Here's how the part is built. I have some questions about the finished solid (model axes, mm). A direction names the side the tool comes from. Coordinates: 2 decimals unless noted, no trailing zeros. Write each loop counter-clockwise with the first axis right and the second up, starting at its lowest first coordinate (ties: lowest second). Pieces come first, ordered by that corner, then holes.
(1) Thinking about a two-plate mould opening in Z: for faces 1 (the flat face through (5, -28, 18)), 2 (the cylindrical face through (9.9, -75, 0.5)), 3 (the flat face through (30, 1, 1)), which applies, released by +Z, released by -Z, zero draft, split by the parting line, or undercut?
(2) Imagine slicing it at A-A, the plane z = 0. List the corners of the cut face in (x, y) for me, plus the area to 3 significant figures.
(3) Imagine slicing it at B-B, the plane x = 27.25. List the corners of the cut face in (y, z) for me, plus the area to 3 significant figures.
(4) For pin 1 Ø10 at (x, z) = (10.5, 45.5) entering from +Y; pin 2 Ø9.5 at (x, z) = (11.5, -34.5) entering from +Y; pin 3 Ø7 at (y, z) = (2.5, 36) entering from +X; pin 4 Ø9 at (y, z) = (-58, 0) entering from -X, each with a flat end and sliding along its axis, tell me the tip position at first contact or that it passes through.
(5) Imagine slicing it at C-C, the plane x = 2. List the corners of the cut face in (y, z) for me, plus the area to 3 significant figures.
(6) Which directions (+Z, -Z, +X, -X, +Y, -Y) give clear straight access to the entire face, cutting with the end or side of a thin tool? Please do faces 4 (the cylindrical face through (9.86, -59.44, 32.58)), 5 (the cylindrical face through (19.86, 20.17, 34.54)), 6 (the cylindrical face through (25, -40, 0)), 7 (the flat face through (17, -7, -31)).
(7) Please list where these lines run through material, in increasing order: probe 1 along Y at (x, z) = (12.25, 0); probe 2 along Y at (x, z) = (8.25, 34.5); probe 3 along Y at (x, z) = (8, -31.5).
(8) Imagine slicing it at D-D, the plane z = -31.5. List the corners of the cut face in (x, y) for me, plus the area to 3 significant figures.
```python
from build123d import *

# Parameters (mm, degrees)
BOSS_EXTRUDE1_DEPTH                             = 10
BOSS_EXTRUDE1_2_DEPTH                           = 10
BOSS_EXTRUDE2_DEPTH                             = 30
BOSS_EXTRUDE3_DEPTH                             = 5
SKETCH1_5_R                                     = 5
BOSS_EXTRUDE4_DEPTH                             = 20
CSK_FOR_M8_FLAT_HEAD_MACHINE_SCREW1_D           = 10
CSK_FOR_M8_FLAT_HEAD_MACHINE_SCREW1_CSINK_D     = 17.3
CSK_FOR_M8_FLAT_HEAD_MACHINE_SCREW1_CSINK_ANGLE = 90


with BuildPart() as part:
    # Sketch1 → Boss-Extrude1 (new body)
    with BuildSketch(Plane(origin=(0, 0, 0), x_dir=(0, 0, -1), z_dir=(1, 0, 0))):
        with BuildLine():
            ThreePointArc((-26.062177826, 31.141016151), (-26.761480784, 36.452749467), (-23.5, 40.703193978))
            Line((-23.5, 40.703193978), (-25.5, 44.167295593))
            ThreePointArc((-25.5, 44.167295593), (-35.403493203, 43.212233307), (-42.62357008, 50.057802056))
            ThreePointArc((-42.62357008, 50.057802056), (-42.094968285, 33.486802939), (-52.43535512, 20.527102646))
            ThreePointArc((-52.43535512, 20.527102646), (-64, 0), (-52.43535512, -20.527102646))
            ThreePointArc((-52.43535512, -20.527102646), (-42.094968285, -33.486802939), (-42.62357008, -50.057802056))
            ThreePointArc((-42.62357008, -50.057802056), (-35.403493203, -43.212233307), (-25.5, -44.167295593))
            Line((-25.5, -44.167295593), (-23.5, -40.703193978))
            ThreePointArc((-23.5, -40.703193978), (-26.761480784, -36.452749467), (-26.062177826, -31.141016151))
            Line((-26.062177826, -31.141016151), (-25.753546494, -30.606451003))
            ThreePointArc((-25.753546494, -30.606451003), (-34.641016151, -20), (-39.382737335, -7))
            Line((-39.382737335, -7), (-40, -7))
            ThreePointArc((-40, -7), (-47, 0), (-40, 7))
            Line((-40, 7), (-39.382737335, 7))
            ThreePointArc((-39.382737335, 7), (-34.641016151, 20), (-25.753546494, 30.606451003))
            Line((-25.753546494, 30.606451003), (-26.062177826, 31.141016151))
        make_face()
    extrude(amount=BOSS_EXTRUDE1_DEPTH)



with BuildPart() as body_2:
    # Sketch1 → Boss-Extrude1 2 (new body)
    with BuildSketch(Plane(origin=(0, 0, 0), x_dir=(0, 0, -1), z_dir=(1, 0, 0))):
        with BuildLine():
            ThreePointArc((25.753546494, 30.606451003), (34.641016151, 20), (39.382737335, 7))
            Line((39.382737335, 7), (40, 7))
            ThreePointArc((40, 7), (47, 0), (40, -7))
            Line((40, -7), (39.382737335, -7))
            ThreePointArc((39.382737335, -7), (34.641016151, -20), (25.753546494, -30.606451003))
            Line((25.753546494, -30.606451003), (26.062177826, -31.141016151))
            ThreePointArc((26.062177826, -31.141016151), (26.761480784, -36.452749467), (23.5, -40.703193978))
            Line((23.5, -40.703193978), (25.5, -44.167295593))
            ThreePointArc((25.5, -44.167295593), (35.403493203, -43.212233307), (42.62357008, -50.057802056))
            ThreePointArc((42.62357008, -50.057802056), (42.094968285, -33.486802939), (52.43535512, -20.527102646))
            ThreePointArc((52.43535512, -20.527102646), (64, 0), (52.43535512, 20.527102646))
            ThreePointArc((52.43535512, 20.527102646), (42.094968285, 33.486802939), (42.62357008, 50.057802056))
            ThreePointArc((42.62357008, 50.057802056), (35.403493203, 43.212233307), (25.5, 44.167295593))
            Line((25.5, 44.167295593), (23.5, 40.703193978))
            ThreePointArc((23.5, 40.703193978), (26.761480784, 36.452749467), (26.062177826, 31.141016151))
            Line((26.062177826, 31.141016151), (25.753546494, 30.606451003))
        make_face()
    extrude(amount=BOSS_EXTRUDE1_2_DEPTH)


with BuildPart() as part_1:
    add(part.part)

    add(body_2.part)  # Boss-Extrude2 merges body 2
    # Sketch1_3 → Boss-Extrude2 (add)
    with BuildSketch(Plane(origin=(0, 0, 0), x_dir=(0, 0, -1), z_dir=(1, 0, 0))):
        with BuildLine():
            Line((21, -7), (21, 7))
            Line((21, 7), (39.382737335, 7))
            ThreePointArc((39.382737335, 7), (34.641016151, 20), (25.753546494, 30.606451003))
            Line((25.753546494, 30.606451003), (16.562177826, 14.686533479))
            Line((16.562177826, 14.686533479), (4.437822174, 21.686533479))
            Line((4.437822174, 21.686533479), (13.629190841, 37.606451003))
            ThreePointArc((13.629190841, 37.606451003), (0, 40), (-13.629190841, 37.606451003))
            Line((-13.629190841, 37.606451003), (-4.437822174, 21.686533479))
            Line((-4.437822174, 21.686533479), (-16.562177826, 14.686533479))
            Line((-16.562177826, 14.686533479), (-25.753546494, 30.606451003))
            ThreePointArc((-25.753546494, 30.606451003), (-34.641016151, 20), (-39.382737335, 7))
            Line((-39.382737335, 7), (-21, 7))
            Line((-21, 7), (-21, -7))
            Line((-21, -7), (-39.382737335, -7))
            ThreePointArc((-39.382737335, -7), (-34.641016151, -20), (-25.753546494, -30.606451003))
            Line((-25.753546494, -30.606451003), (-16.562177826, -14.686533479))
            Line((-16.562177826, -14.686533479), (-4.437822174, -21.686533479))
            Line((-4.437822174, -21.686533479), (-13.629190841, -37.606451003))
            ThreePointArc((-13.629190841, -37.606451003), (0, -40), (13.629190841, -37.606451003))
            Line((13.629190841, -37.606451003), (4.437822174, -21.686533479))
            Line((4.437822174, -21.686533479), (16.562177826, -14.686533479))
            Line((16.562177826, -14.686533479), (25.753546494, -30.606451003))
            ThreePointArc((25.753546494, -30.606451003), (34.641016151, -20), (39.382737335, -7))
            Line((39.382737335, -7), (21, -7))
        make_face()
    extrude(amount=BOSS_EXTRUDE2_DEPTH)

    # Sketch1_4 → Boss-Extrude3 (add)
    with BuildSketch(Plane(origin=(0, 0, 0), x_dir=(0, 0, -1), z_dir=(1, 0, 0))):
        with BuildLine():
            ThreePointArc((13.937822174, 38.141016151), (23.5, 40.703193978), (26.062177826, 31.141016151))
            Line((26.062177826, 31.141016151), (16.562177826, 14.686533479))
            Line((16.562177826, 14.686533479), (4.437822174, 21.686533479))
            Line((4.437822174, 21.686533479), (13.937822174, 38.141016151))
        make_face()
        with BuildLine():
            ThreePointArc((-26.062177826, 31.141016151), (-23.5, 40.703193978), (-13.937822174, 38.141016151))
            Line((-13.937822174, 38.141016151), (-4.437822174, 21.686533479))
            Line((-4.437822174, 21.686533479), (-16.562177826, 14.686533479))
            Line((-16.562177826, 14.686533479), (-26.062177826, 31.141016151))
        make_face()
        with BuildLine():
            ThreePointArc((40, 7), (47, 0), (40, -7))
            Line((40, -7), (21, -7))
            Line((21, -7), (21, 7))
            Line((21, 7), (40, 7))
        make_face()
        with BuildLine():
            ThreePointArc((-40, -7), (-47, 0), (-40, 7))
            Line((-40, 7), (-21, 7))
            Line((-21, 7), (-21, -7))
            Line((-21, -7), (-40, -7))
        make_face()
        with BuildLine():
            ThreePointArc((-13.937822174, -38.141016151), (-23.5, -40.703193978), (-26.062177826, -31.141016151))
            Line((-26.062177826, -31.141016151), (-16.562177826, -14.686533479))
            Line((-16.562177826, -14.686533479), (-4.437822174, -21.686533479))
            Line((-4.437822174, -21.686533479), (-13.937822174, -38.141016151))
        make_face()
        with BuildLine():
            ThreePointArc((26.062177826, -31.141016151), (23.5, -40.703193978), (13.937822174, -38.141016151))
            Line((13.937822174, -38.141016151), (4.437822174, -21.686533479))
            Line((4.437822174, -21.686533479), (16.562177826, -14.686533479))
            Line((16.562177826, -14.686533479), (26.062177826, -31.141016151))
        make_face()
    extrude(amount=BOSS_EXTRUDE3_DEPTH)

    # Sketch1_5 → Boss-Extrude4 (add)
    # profile 1 of 2: a face of its own
    with BuildSketch(Plane(origin=(0, 0, 0), x_dir=(0, 0, -1), z_dir=(1, 0, 0))):
        with BuildLine():
            ThreePointArc((13.937822174, 38.141016151), (18.188266684, 41.402496935), (23.5, 40.703193978))
            Line((23.5, 40.703193978), (25.5, 44.167295593))
            ThreePointArc((25.5, 44.167295593), (35.403493203, 43.212233307), (42.62357008, 50.057802056))
            ThreePointArc((42.62357008, 50.057802056), (42.847367131, 58.463093642), (37.5, 64.951905284))
            ThreePointArc((37.5, 64.951905284), (0, 75), (-37.5, 64.951905284))
            ThreePointArc((-37.5, 64.951905284), (-42.847367131, 58.463093642), (-42.62357008, 50.057802056))
            ThreePointArc((-42.62357008, 50.057802056), (-35.403493203, 43.212233307), (-25.5, 44.167295593))
            Line((-25.5, 44.167295593), (-23.5, 40.703193978))
            ThreePointArc((-23.5, 40.703193978), (-18.188266684, 41.402496935), (-13.937822174, 38.141016151))
            Line((-13.937822174, 38.141016151), (-13.629190841, 37.606451003))
            ThreePointArc((-13.629190841, 37.606451003), (0, 40), (13.629190841, 37.606451003))
            Line((13.629190841, 37.606451003), (13.937822174, 38.141016151))
        make_face()
        with Locations((-31.5, 54.559600438)):
            Circle(SKETCH1_5_R, mode=Mode.SUBTRACT)
        with Locations((31.5, 54.559600438)):
            Circle(SKETCH1_5_R, mode=Mode.SUBTRACT)
        with Locations((0, 58)):
            Circle(SKETCH1_5_R, mode=Mode.SUBTRACT)
    # profile 2 of 2: a face of its own
    with BuildSketch(Plane(origin=(0, 0, 0), x_dir=(0, 0, -1), z_dir=(1, 0, 0))):
        with BuildLine():
            Line((25.5, -44.167295593), (23.5, -40.703193978))
            ThreePointArc((23.5, -40.703193978), (18.188266684, -41.402496935), (13.937822174, -38.141016151))
            Line((13.937822174, -38.141016151), (13.629190841, -37.606451003))
            ThreePointArc((13.629190841, -37.606451003), (0, -40), (-13.629190841, -37.606451003))
            Line((-13.629190841, -37.606451003), (-13.937822174, -38.141016151))
            ThreePointArc((-13.937822174, -38.141016151), (-18.188266684, -41.402496935), (-23.5, -40.703193978))
            Line((-23.5, -40.703193978), (-25.5, -44.167295593))
            ThreePointArc((-25.5, -44.167295593), (-35.403493203, -43.212233307), (-42.62357008, -50.057802056))
            ThreePointArc((-42.62357008, -50.057802056), (-42.847367131, -58.463093642), (-37.5, -64.951905284))
            ThreePointArc((-37.5, -64.951905284), (0, -75), (37.5, -64.951905284))
            ThreePointArc((37.5, -64.951905284), (42.847367131, -58.463093642), (42.62357008, -50.057802056))
            ThreePointArc((42.62357008, -50.057802056), (35.403493203, -43.212233307), (25.5, -44.167295593))
        make_face()
        with Locations((-31.5, -54.559600438)):
            Circle(SKETCH1_5_R, mode=Mode.SUBTRACT)
        with Locations((0, -58)):
            Circle(SKETCH1_5_R, mode=Mode.SUBTRACT)
        with Locations((31.5, -54.559600438)):
            Circle(SKETCH1_5_R, mode=Mode.SUBTRACT)
    extrude(amount=BOSS_EXTRUDE4_DEPTH)

    # CSK for M8 Flat Head Machine Screw1 (through all)
    with Locations(Plane(origin=(20, 0, 0), x_dir=(0, 0, -1), z_dir=(1, 0, 0))):
        with Locations((0, 58), (0, -58)):
            CounterSinkHole(CSK_FOR_M8_FLAT_HEAD_MACHINE_SCREW1_D / 2, CSK_FOR_M8_FLAT_HEAD_MACHINE_SCREW1_CSINK_D / 2, counter_sink_angle=CSK_FOR_M8_FLAT_HEAD_MACHINE_SCREW1_CSINK_ANGLE)


solid = part_1.part
```
Recorded:
1. face 1: undercut
1. face 2: split by the parting line
1. face 3: zero draft
2. outline: (0, -75) - (20, -75) - (20, -66.65) - (16.35, -63) - (0, -63) - close; (0, -53) - (16.35, -53) - (20, -49.35) - (20, -40) - (30, -40) - (30, 40) - (20, 40) - (20, 49.35) - (16.35, 53) - (0, 53) - close; (0, 63) - (16.35, 63) - (20, 66.65) - (20, 75) - (0, 75) - close
2. area: 3,370 mm2
3. outline: (-37.61, -13.63) - (-21.69, -4.44) - (-14.69, -16.56) - (-30.61, -25.75) arc R40 ccw to (-7, -39.38) - (-7, -21) - (7, -21) - (7, -39.38) arc R40 ccw to (30.61, -25.75) - (14.69, -16.56) - (21.69, -4.44) - (37.61, -13.63) arc R40 ccw to (37.61, 13.63) - (21.69, 4.44) - (14.69, 16.56) - (30.61, 25.75) arc R40 ccw to (7, 39.38) - (7, 21) - (-7, 21) - (-7, 39.38) arc R40 ccw to (-30.61, 25.75) - (-14.69, 16.56) - (-21.69, 4.44) - (-37.61, 13.63) arc R40 ccw to start
3. area: 3,450 mm2
4. pin 1: stops at y = 62.5
4. pin 2: stops at y = 68.85
4. pin 3: stops at x = 5
4. pin 4: passes through
5. outline: (-64.95, -37.5) arc R12 ccw to (-50.06, -42.62) arc R24 cw to (-20.53, -52.44) arc R24 ccw to (20.53, -52.44) arc R24 cw to (50.06, -42.62) arc R12 ccw to (64.95, -37.5) arc R75 ccw to (64.95, 37.5) arc R12 ccw to (50.06, 42.62) arc R24 cw to (20.53, 52.44) arc R24 ccw to (-20.53, 52.44) arc R24 cw to (-50.06, 42.62) arc R12 ccw to (-64.95, 37.5) arc R75 ccw to start; hole circle Ø10 at (-58, 0); hole circle Ø10 at (-54.56, -31.5); hole circle Ø10 at (-54.56, 31.5); hole circle Ø10 at (54.56, -31.5); hole circle Ø10 at (54.56, 31.5); hole circle Ø10 at (58, 0)
5. area: 13,200 mm2
6. face 4: +X, -X
6. face 5: +Z, +X
6. face 6: +X, -Y
6. face 7: +X
7. probe 1: y = -75 to -63, -53 to 53, 63 to 75
7. probe 2: y = -66.59 to -58.56, -50.56 to -7, 7 to 50.56, 58.56 to 66.59
7. probe 3: y = -68.06 to -59.56, -49.56 to -7, 7 to 49.56, 59.56 to 68.06
8. outline: (0, -68.06) - (20, -68.06) - (20, -59.56) - (0, -59.56) - close; (0, -49.56) - (20, -49.56) - (20, -42.56) - (10, -42.56) - (10, -24.65) - (30, -24.65) - (30, -7) - (5, -7) - (5, 7) - (30, 7) - (30, 24.65) - (10, 24.65) - (10, 42.56) - (20, 42.56) - (20, 49.56) - (0, 49.56) - close; (0, 59.56) - (20, 59.56) - (20, 68.06) - (0, 68.06) - close
8. area: 2,110 mm2
